Geometry check sheet. Reference: the model listing, model coordinates, mm. A direction names the side the tool comes from. Give positions to 0.01 mm unless a question says otherwise; leave off trailing zeros. Write each loop counter-clockwise with the first axis right and the second up, starting at its lowest first coordinate (ties: lowest second). Pieces come first, ordered by that corner, then holes. Notation, with made-up numbers: (10.25, 3.5) - (27.25, 3.5) arc R18 ccw to (27.25, 16.5) - close; hole circle Ø5 at (80.5, 25). An arc over 180 degrees is marked (long way). Write item = value, one per line. Start each with the question number.
(1) Section check B-B, the plane x = 8. Enter the section's corners in (y, z).
(2) Section check A-A, the plane y = -12. Enter the section's corners in (x, z).
(3) Section check C-C, the plane y = -26.5. Enter the section's corners in (x, z), plus the area to 3 significant figures.
(4) Thickness scan on L1, parallel to Y at x = -44.8, z = -10.5; L2, parallel to Y at x = -44.1, z = 10.5; L3, parallel to Y at x = -27.5, z = 0. Record the ranges inside material, lowest first.
(5) Section check D-D, the plane z = 2.5. Enter the section's corners in (x, y), plus the area to 3 significant figures.
(6) Depth check by flat-ended pin: pin 1 Ø0.9 at (y, z) = (-38, -10.5) entering from -X. Enter the tip coordinate at first touch or a pass-through.
(7) Draft check along Y on faces 1 (the flat face through (-45.15, 1, 0)), 2 (the flat face through (25, -44.25, 0)), 3 (the cylindrical face through (43.037, -42.098, -11.556)). Enter one of: pulls with the +Y half, pulls with the -Y half, needs draft (parallel to the pull), parting line crosses it, or undercut.
(8) Access from +Z, -Z, +X, -X, +Y, -Y to the whole of each face (thin tool, end or side, straight path). Record for faces 4 (the cylindrical face through (44.194, -36.036, -10.175)), 5 (the cylindrical face through (43.037, 42.098, 11.556)), 6 (the flat face through (19.6, 41.5, -7.5)), 7 (the flat face through (0, 43.55, 0)), 8 (the flat face through (42.15, 1, 0)).
Autodesk Inventor part; units mm, degrees
ref_plane "YZ Plane" through (0, 0, 0) normal (1, 0, 0) x (0, 1, 0)
ref_plane "XZ Plane" through (0, 0, 0) normal (0, 1, 0) x (-1, 0, 0)
ref_plane "XY Plane" through (0, 0, 0) normal (0, 0, 1) x (1, 0, 0)
sketch "Sketch1" plane through (0, 0, 0) normal (0, 0, 1) x (1, 0, 0)
  line L0 (-45.15, -44.25) -> (45.15, -44.25)
  line L1 (45.15, -44.25) -> (45.15, 44.25)
  line L2 (45.15, 44.25) -> (-45.15, 44.25)
  line L3 (-45.15, 44.25) -> (-45.15, -44.25)
  line L4 (-45.15, -44.25) -> (45.15, 44.25) construction
  line L5 (45.15, -44.25) -> (-45.15, 44.25) construction
  line L6 (42.15, -41.25) -> (-42.15, -41.25)
  line L7 (-42.15, -41.25) -> (-42.15, 41.25)
  line L8 (-42.15, 41.25) -> (42.15, 41.25)
  line L9 (42.15, 41.25) -> (42.15, -41.25)
  line L10 (42.15, -41.25) -> (-42.15, 41.25) construction
  line L11 (-42.15, -41.25) -> (42.15, 41.25) construction
  point P0 (0, 0)
  dimension "d0" = 90.3
  dimension "d1" = 88.5
  dimension "d2" = 84.3
  dimension "d3" = 82.5
extrude "Extrusion1" add sketch "Sketch1" along normal mid plane 31
sketch "Sketch2" plane through (0, 0, -15.5) normal (0, 0, -1) x (-1, 0, 0)
  line L0 (42.15, 41.25) -> (42.15, -41.25)
  line L1 (42.15, -41.25) -> (-42.15, -41.25)
  line L2 (-42.15, -41.25) -> (-42.15, 41.25)
  line L3 (-42.15, 41.25) -> (42.15, 41.25)
  line L4 (41.25, -42.85) -> (-41.25, -42.85)
  line L5 (-43.75, -40.35) -> (-43.75, 40.35)
  line L6 (-41.25, 42.85) -> (41.25, 42.85)
  line L7 (43.75, 40.35) -> (43.75, -40.35)
  line L8 (43.75, -42.85) -> (-43.75, 42.85) construction
  line L9 (-43.75, -42.85) -> (43.75, 42.85) construction
  arc A0 (-41.25, 42.85) -> (-43.75, 40.35) centre (-41.25, 40.35) ccw
  arc A1 (-43.75, -40.35) -> (-41.25, -42.85) centre (-41.25, -40.35) ccw
  arc A2 (41.25, -42.85) -> (43.75, -40.35) centre (41.25, -40.35) ccw
  arc A3 (43.75, 40.35) -> (41.25, 42.85) centre (41.25, 40.35) ccw
  point P0 (0, 0)
  dimension "d8" = 2.5
  dimension "d40" = 1.6
  dimension "d41" = 1.6
extrude "Extrusion2" cut sketch "Sketch2" against normal blind 8
mirror "Mirror1" about plane through (0, 0, 0) normal (0, 0, 1) of "Extrusion2"
sketch "Sketch3" plane through (-45.15, -44.25, 15.5) normal (-1, 0, 0) x (0, -1, 0)
  line L0 (0, 0) -> (0, -31)
  line L1 (-9, -26.4) -> (-9, -20.4)
  line L2 (-10, -19.4) -> (-28, -19.4)
  line L3 (-29, -20.4) -> (-29, -26.4)
  arc A0 (-28, -19.4) -> (-29, -20.4) centre (-28, -20.4) ccw
  arc A1 (-9, -20.4) -> (-10, -19.4) centre (-10, -20.4) ccw
  line L4 (-29, -26.4) -> (-9, -26.4)
  line L5 (0, -31) -> (-88.5, -31)
  point P0 (-44.25, -15.5)
  dimension "d11" = 1
  dimension "d12" = 20
  dimension "d44" = 7
  dimension "d45" = 4.6
  dimension "d47" = 29
extrude "Elect" cut sketch "Sketch3" against normal blind 5
sketch "Sketch5" plane through (-45.15, -44.25, 15.5) normal (-1, 0, 0) x (0, 0, 1)
  line L0 (-31, 88.5) -> (0, 88.5)
  line L1 (-31, 0) -> (-31, 88.5)
  line L2 (-13.5, 72.7) -> (-10, 72.7)
  line L3 (-10, 72.7) -> (-10, 65.5)
  line L4 (-10, 65.5) -> (-13.5, 65.5)
  line L5 (-13.5, 65.5) -> (-13.5, 72.7)
  point P0 (-15.5, 44.25)
  point P1 (-11.75, 72.7)
  point P2 (-13.5, 69.1)
  dimension "d23" = 3.5
  dimension "d24" = 7.2
  dimension "d42" = 21
  dimension "d43" = 23
extrude "Mini-usb" cut sketch "Sketch5" against normal blind 10
sketch "Sketch7" plane through (-45.15, -44.25, 15.5) normal (-1, 0, 0) x (0, 0, 1)
  line L0 (-13.5, 65.5) -> (-13.5, 72.7)
  line L1 (-10, 72.7) -> (-10, 65.5)
  line L2 (-10, 65.5) -> (-13.5, 65.5)
  line L3 (-10, 72.7) -> (-13.5, 72.7)
  line L4 (-10, 72.7) -> (-13.5, 65.5) construction
  line L5 (-13.5, 65.5) -> (-10, 65.5)
  line L6 (-10, 65.5) -> (-13.5, 72.7) construction
  line L7 (-15.25, 75.1) -> (-8.25, 75.1)
  line L8 (-7.25, 74.1) -> (-7.25, 64.1)
  line L9 (-8.25, 63.1) -> (-15.25, 63.1)
  line L10 (-16.25, 64.1) -> (-16.25, 74.1)
  line L11 (-16.25, 75.1) -> (-7.25, 63.1) construction
  line L12 (-7.25, 75.1) -> (-16.25, 63.1) construction
  arc A0 (-7.25, 74.1) -> (-8.25, 75.1) centre (-8.25, 74.1) ccw
  arc A1 (-15.25, 75.1) -> (-16.25, 74.1) centre (-15.25, 74.1) ccw
  arc A2 (-16.25, 64.1) -> (-15.25, 63.1) centre (-15.25, 64.1) ccw
  arc A3 (-8.25, 63.1) -> (-7.25, 64.1) centre (-8.25, 64.1) ccw
  point P0 (-15.5, 44.25)
  point P1 (-11.75, 69.1)
  dimension "d35" = 12
  dimension "d36" = 9
  dimension "d37" = 1
extrude "USB" cut sketch "Sketch7" against normal blind 3
sketch "Sketch6" plane through (0, 0, 15.5) normal (0, 0, 1) x (1, 0, 0)
  line L0 (45.15, 44.25) -> (-45.15, 44.25)
  line L1 (-5, 44.25) -> (5, 44.25)
  line L2 (5, 44.25) -> (5, 43.55)
  line L3 (5, 43.55) -> (-5, 43.55)
  line L4 (-5, 43.55) -> (-5, 44.25)
  point P0 (0, 0)
  point P1 (0, 43.55)
  dimension "d31" = 10
  dimension "d32" = 0.7
extrude "Decoratie" cut sketch "Sketch6" against normal through all
mirror "Mirror2" about plane through (0, 0, 0) normal (0, 1, 0) of "Decoratie"
fillet "Fillet1" radius 1 4 edges at (42.15, 41.25, 0) (-42.15, 41.25, 0) (-42.15, -41.25, 0) (42.15, -41.25, 0)
sketch "Sketch8" plane through (45.15, -44.25, 15.5) normal (1, 0, 0) x (0, 0, -1)
  circle A0 centre (5, 6.75) radius 0.65
  circle A1 centre (5, 81.75) radius 0.65
  line L0 (0, 0) -> (0, 88.5)
  line L1 (5, 6.75) -> (5, 81.75) construction
  circle A2 centre (26, 6.75) radius 0.65
  circle A3 centre (26, 81.75) radius 0.65
  line L2 (31, 88.5) -> (31, 0)
  point P0 (15.5, 44.25)
  point P1 (5, 44.25)
  dimension "d49" = 1.3
  dimension "d51" = 75
  dimension "d52" = 5
  dimension "d55" = 5
extrude "Extrusion8" cut sketch "Sketch8" against normal through all
sketch "Sketch9" plane through (-43.75, -40.35, 15.5) normal (1, 0, 0) x (0, 0, -1)
  circle A0 centre (5, 2.85) radius 0.65
  circle A1 centre (26, 2.85) radius 0.65
  circle A2 centre (26, 77.85) radius 0.65
  circle A3 centre (5, 77.85) radius 0.65
  circle A4 centre (5, 77.85) radius 1.5
  circle A5 centre (5, 2.85) radius 1.5
  circle A6 centre (26, 2.85) radius 1.5
  circle A7 centre (26, 77.85) radius 1.5
  point P0 (15.5, 40.35)
  dimension "d58" = 3
  dimension "d59" = 3
  dimension "d60" = 3
  dimension "d61" = 3
extrude "Extrusion9" cut sketch "Sketch9" against normal blind 0.9
mirror "Mirror3" about plane through (0, 0, 0) normal (1, 0, 0) of "Extrusion9"
properties part number "AP-02" material "Q235"
Model answer:
q1.outline = (-44.25, -15.5) - (-42.85, -15.5) - (-42.85, -7.5) - (-41.25, -7.5) - (-41.25, 7.5) - (-42.85, 7.5) - (-42.85, 15.5) - (-44.25, 15.5) - close; (41.25, -7.5) - (42.85, -7.5) - (42.85, -15.5) - (44.25, -15.5) - (44.25, 15.5) - (42.85, 15.5) - (42.85, 7.5) - (41.25, 7.5) - close
q2.outline = (-45.15, -15.5) - (-43.75, -15.5) - (-43.75, -7.5) - (-42.15, -7.5) - (-42.15, 7.5) - (-43.75, 7.5) - (-43.75, 15.5) - (-45.15, 15.5) - close; (42.15, -7.5) - (43.75, -7.5) - (43.75, -15.5) - (45.15, -15.5) - (45.15, 15.5) - (43.75, 15.5) - (43.75, 7.5) - (42.15, 7.5) - close
q3.outline = (-45.15, -15.5) - (-43.75, -15.5) - (-43.75, -10.9) - (-45.15, -10.9) - close; (-45.15, -3.9) - (-42.15, -3.9) - (-42.15, 7.5) - (-43.75, 7.5) - (-43.75, 15.5) - (-45.15, 15.5) - close; (42.15, -7.5) - (43.75, -7.5) - (43.75, -15.5) - (45.15, -15.5) - (45.15, 15.5) - (43.75, 15.5) - (43.75, 7.5) - (42.15, 7.5) - close
q3.area = 119 mm²
q4.L1 = -44.25 to -38.15, -36.85 to -35.25, -15.25 to 36.85, 38.15 to 44.25
q4.L2 = -44.25 to -39, -36 to 36, 39 to 44.25
q4.L3 = -44.25 to -41.25, 41.25 to 44.25
q5.outline = (-45.15, -44.25) - (-5, -44.25) - (-5, -43.55) - (5, -43.55) - (5, -44.25) - (45.15, -44.25) - (45.15, 44.25) - (5, 44.25) - (5, 43.55) - (-5, 43.55) - (-5, 44.25) - (-45.15, 44.25) - (-45.15, 30.85) - (-42.15, 30.85) - (-42.15, 40.25) arc R1 cw to (-41.15, 41.25) - (41.15, 41.25) arc R1 cw to (42.15, 40.25) - (42.15, -40.25) arc R1 cw to (41.15, -41.25) - (-41.15, -41.25) arc R1 cw to (-42.15, -40.25) - (-42.15, 18.85) - (-45.15, 18.85) - close
q5.area = 988 mm²
q6.pin_1 = -45.15
q7.face_1 = needs draft
q7.face_2 = pulls with the -Y half
q7.face_3 = undercut
q8.face_4 = none
q8.face_5 = +Z
q8.face_6 = -Z
q8.face_7 = +Z, -Z, +Y
q8.face_8 = +Z, -Z
